from build123d import *

# Parameters (mm, degrees)
EXTRUDE_1_DEPTH     = 3
SKETCH_3_R          = 2.5
SKETCH_3_R_2        = 2.1
CUT_EXTRUDE_1_DEPTH = 61.517481152
SKETCH_4_R          = 2
CUT_EXTRUDE_2_DEPTH = 10


with BuildPart() as part:
    # 草图2 → 凸台-拉伸1 (new body)
    with BuildSketch(Plane.XY):
        Polygon((32.5, 23.375), (-32.5, 23.375), (-32.5, 27.675), (-37.93, 27.675), (-37.93, 36.825), (-47.93, 36.825), (-47.93, 15.805), (-35.97, 15.805), (-35.97, -28.325), (-37.47, -28.325), (-37.47, -36.825), (-9.97, -36.825), (-9.97, -17.825), (9.97, -17.825), (9.97, -36.825), (37.47, -36.825), (37.47, -28.325), (35.97, -28.325), (35.97, 15.805), (47.93, 15.805), (47.93, 36.825), (37.93, 36.825), (37.93, 27.675), (32.5, 27.675), align=None)
    extrude(amount=EXTRUDE_1_DEPTH)

    # 草图3 → 切除-拉伸1 (cut, through all)
    with BuildSketch(Plane.XY.offset(3)):
        with Locations((-28, 19.875)):
            Circle(SKETCH_3_R)
        with Locations((-13.5, -29.625)):
            Circle(SKETCH_3_R_2)
        with Locations(Location((13.5, -29.625, 0), (0, 0, 180))):
            Circle(SKETCH_3_R_2)
        with Locations(Location((28, 19.875, 0), (0, 0, 180))):
            Circle(SKETCH_3_R)
    extrude(amount=-CUT_EXTRUDE_1_DEPTH, mode=Mode.SUBTRACT)

    # 草图4 → 切除-拉伸2 (cut)
    with BuildSketch(Plane.XY.offset(3)):
        with Locations((-42, 33)):
            Circle(SKETCH_4_R)
        with Locations((-30, -33)):
            Circle(SKETCH_4_R)
        with Locations((30, -33)):
            Circle(SKETCH_4_R)
        with Locations((42, 33)):
            Circle(SKETCH_4_R)
    extrude(amount=-CUT_EXTRUDE_2_DEPTH, mode=Mode.SUBTRACT)


solid = part.part
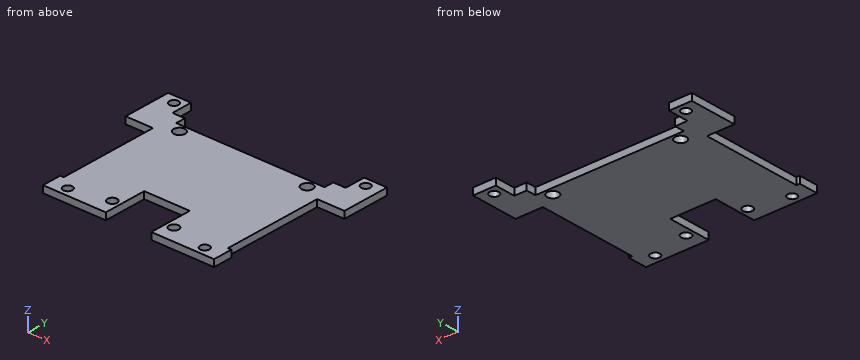
The model under review builds one solid part; all positions refer to its coordinate system, in mm. Round coordinates to 2 decimals unless told otherwise and drop trailing zeros. Loops run counter-clockwise (first coordinate to the right, second up) from the corner with the lowest first, then second, coordinate; pieces in that order, holes last. Notation, with made-up numbers: (84, 78) -> (114, 78) arc R27 cw to (114, 95) -> close; hole circle Ø9 at (41, 79). An arc over 180 degrees is marked (long way). Return JSON: item names as keys, results as strings.
(1) Add section B-B on x = 13.5. Write out the cut boundary in (y, z) (3 decimals), plus the area to 3 significant figures.
Solved:
{"outline": "(-36.825, 0) -> (-31.725, 0) -> (-31.725, 3) -> (-36.825, 3) -> close; (-27.525, 0) -> (23.375, 0) -> (23.375, 3) -> (-27.525, 3) -> close", "area": "168 mm2"}
(2) Add section D-D on z = 2.2. State how many separate pieces and enclosed holes the cut face has, plus the area to 3 significant figures.
Solved:
{"separate pieces": "1", "enclosed holes": "8", "area": "4,360 mm2"}
(3) For line 1 (X direction, y = -21.5, z = 2.8); line 2 (X direction, y = -29.5, z = 0.2); line 3 (Y direction, x = 37, z = 0.45) (3 decimals), list the stretches that pass through material, from the lowest coordinate up.
Solved:
{"line 1": "-35.97 to -9.97, 9.97 to 35.97", "line 2": "-37.47 to -15.6, -11.4 to -9.97, 9.97 to 11.4, 15.6 to 37.47", "line 3": "-36.825 to -28.325, 15.805 to 27.675"}
(4) Add section A-A on y = 33. Write out the cut boundary in (x, z).
Solved:
{"outline": "(-47.93, 0) -> (-44, 0) -> (-44, 3) -> (-47.93, 3) -> close; (-40, 0) -> (-37.93, 0) -> (-37.93, 3) -> (-40, 3) -> close; (37.93, 0) -> (40, 0) -> (40, 3) -> (37.93, 3) -> close; (44, 0) -> (47.93, 0) -> (47.93, 3) -> (44, 3) -> close"}
(5) Add section C-C on y = -26. Write out the cut boundary in (x, z).
Solved:
{"outline": "(-35.97, 0) -> (-9.97, 0) -> (-9.97, 3) -> (-35.97, 3) -> close; (9.97, 0) -> (35.97, 0) -> (35.97, 3) -> (9.97, 3) -> close"}
(6) For pin 1 (0.9 mm diameter, centred on y = -1, z = 1.5, fed in from -X); pin 2 (0.9 mm diameter, centred on y = -25, z = 1.5, fed in from +X); pin 3 (1 mm diameter, centred on x = 22, z = 1, fed in from +Y) (3 decimals), all flat-tipped, find the tip position at first contact; note any pin that passes through.
Solved:
{"pin 1": "x = -35.97", "pin 2": "x = 35.97", "pin 3": "y = 23.375"}
